```python
from build123d import *

# Parameters (mm, degrees)
SKETCH1_R           = 1.45
BOSS_EXTRUDE1_DEPTH = 4
SKETCH2_W           = 3
SKETCH2_H           = 51.803847578
SKETCH2_W_2         = 66.803847578
SKETCH2_H_2         = 3
CUT_EXTRUDE1_DEPTH  = 3


with BuildPart() as part:
    # Sketch1 → Boss-Extrude1 (new body)
    with BuildSketch(Plane(origin=(0, 0, 0), x_dir=(1, 0, 0), z_dir=(0, 1, 0))):
        with BuildLine():
            Line((-33.401923789, 30), (33.401923789, 30))
            ThreePointArc((33.401923789, 30), (38.121320344, 30.621320344), (37.5, 25.901923789))
            Line((37.5, 25.901923789), (37.5, -25.901923789))
            ThreePointArc((37.5, -25.901923789), (38.121320344, -30.621320344), (33.401923789, -30))
            Line((33.401923789, -30), (-33.401923789, -30))
            ThreePointArc((-33.401923789, -30), (-38.121320344, -30.621320344), (-37.5, -25.901923789))
            Line((-37.5, -25.901923789), (-37.5, 25.901923789))
            ThreePointArc((-37.5, 25.901923789), (-38.121320344, 30.621320344), (-33.401923789, 30))
        make_face()
        with Locations((36, 28.5)):
            Circle(SKETCH1_R, mode=Mode.SUBTRACT)
        with Locations((36, -28.5)):
            Circle(SKETCH1_R, mode=Mode.SUBTRACT)
        with Locations((-36, -28.5)):
            Circle(SKETCH1_R, mode=Mode.SUBTRACT)
        with Locations((-36, 28.5)):
            Circle(SKETCH1_R, mode=Mode.SUBTRACT)
        with BuildLine():
            Line((-33.401923789, 27), (33.401923789, 27))
            ThreePointArc((33.401923789, 27), (33.878679656, 26.378679656), (34.5, 25.901923789))
            Line((34.5, 25.901923789), (34.5, -25.901923789))
            ThreePointArc((34.5, -25.901923789), (33.878679656, -26.378679656), (33.401923789, -27))
            Line((33.401923789, -27), (-33.401923789, -27))
            ThreePointArc((-33.401923789, -27), (-33.878679656, -26.378679656), (-34.5, -25.901923789))
            Line((-34.5, -25.901923789), (-34.5, 25.901923789))
            ThreePointArc((-34.5, 25.901923789), (-33.878679656, 26.378679656), (-33.401923789, 27))
        make_face(mode=Mode.SUBTRACT)
    extrude(amount=BOSS_EXTRUDE1_DEPTH)

    # Sketch2 → Cut-Extrude1 (cut)
    with BuildSketch(Plane(origin=(0, 4, 0), x_dir=(1, 0, 0), z_dir=(0, 1, 0))):
        with Locations((-36, 0)):
            Rectangle(SKETCH2_W, SKETCH2_H)
        with Locations((0, -28.5)):
            Rectangle(SKETCH2_W_2, SKETCH2_H_2)
        with Locations((36, 0)):
            Rectangle(SKETCH2_W, SKETCH2_H)
        with Locations((0, 28.5)):
            Rectangle(SKETCH2_W_2, SKETCH2_H_2)
    extrude(amount=-CUT_EXTRUDE1_DEPTH, mode=Mode.SUBTRACT)


solid = part.part
```
CAD build for the part. Positions are in the model's coordinates, mm. A direction names the side the tool comes from. Round coordinates to 2 decimals unless told otherwise and drop trailing zeros. Order: outer loops, then holes, each group sorted by start corner. A loop starts at its lowest first (then second) coordinate and runs counter-clockwise, first axis right, second up.
Q1. Slice it at D-D (z = -7). Write the cut outline in (x, y).
Q2. Two-plate mould, pull along X, no slides. Class faces 4 (the flat face through (37.5, 4, -29.4)), 5 (the flat face through (-33.402, 3, -28)): pulls with the +X half, pulls with the -X half, needs draft (parallel to the pull), parting line crosses it, or undercut.
Q3. Drop flat-ended pins along their axis: pin 1 (0.5 mm diameter, centred on x = 3, y = 0.5, fed in from +Z); pin 2 (1.1 mm diameter, centred on x = -3, y = 0.5, fed in from -Z); pin 3 (2.5 mm diameter, centred on x = -2.5, z = 29, fed in from +Y). Give the stop position or say it passes through.
Q4. Wall check: L1, parallel to X at y = 2.7, z = 28.5; L2, parallel to Z at x = 36, y = 1.8; L3, parallel to Z at x = -25, y = 0.6. Give the ranges that are in metal, low to high.
Q5. Which spindle directions (+Z, -Z, +X, -X, +Y, -Y) get a long thin tool onto all of the face, cutting with end or side? Do faces 1 (the flat face through (-36, 1, 0)), 2 (the cylindrical face through (35.686, 1.972, -27.084)), 3 (the flat face through (0, 1, -29)). Say none if no direction does.
Q6. Slice it at C-C (x = 36). Write the cut outline in (y, z), and give its area (3 significant figures).
Q7. Slice it at B-B (y = 3.4). Write the cut outline in (x, z), and give its area (3 significant figures).
Q8. Slice it at A-A (x = -13). Write the cut outline in (y, z).
Results below:
1. outline: (-37.5, 0) - (-34.5, 0) - (-34.5, 1) - (-37.5, 1) - close; (34.5, 0) - (37.5, 0) - (37.5, 1) - (34.5, 1) - close
2. face 4: needs draft
2. face 5: undercut
3. pin 1: stops at z = 30
3. pin 2: stops at z = -30
3. pin 3: stops at y = 1
4. L1: x = -39 to -37.45, -34.55 to -33.4, 33.4 to 34.55, 37.45 to 39
4. L2: z = -31.5 to -29.95, -27.05 to -25.9, 25.9 to 27.05, 29.95 to 31.5
4. L3: z = -30 to -27, 27 to 30
5. face 1: +X, -X, +Y
5. face 2: +Y, -Y
5. face 3: +Z, -Z, +Y
6. outline: (0, -31.5) - (4, -31.5) - (4, -29.95) - (0, -29.95) - close; (0, -27.05) - (4, -27.05) - (4, -25.9) - (1, -25.9) - (1, 25.9) - (4, 25.9) - (4, 27.05) - (0, 27.05) - close; (0, 29.95) - (4, 29.95) - (4, 31.5) - (0, 31.5) - close
6. area: 73.4 mm2
7. outline: (-37.5, -25.9) arc R3 ccw (long way) to (-33.4, -30) - (-33.4, -27) arc R3 ccw to (-34.5, -25.9) - close; (-37.5, 25.9) - (-34.5, 25.9) arc R3 ccw to (-33.4, 27) - (-33.4, 30) arc R3 ccw (long way) to start; (33.4, -30) arc R3 ccw (long way) to (37.5, -25.9) - (34.5, -25.9) arc R3 ccw to (33.4, -27) - close; (33.4, 27) arc R3 ccw to (34.5, 25.9) - (37.5, 25.9) arc R3 ccw (long way) to (33.4, 30) - close; hole circle Ø2.9 at (-36, -28.5); hole circle Ø2.9 at (-36, 28.5); hole circle Ø2.9 at (36, -28.5); hole circle Ø2.9 at (36, 28.5)
7. area: 80.2 mm2
8. outline: (0, -30) - (1, -30) - (1, -27) - (0, -27) - close; (0, 27) - (1, 27) - (1, 30) - (0, 30) - close
